Check sheet for the modelled part. Datum: model origin and axes. Units: mm. A direction names the side the tool comes from. Give positions to 0.01 mm unless a question says otherwise; leave off trailing zeros. Order: outer loops, then holes, each group sorted by start corner. A loop starts at its lowest first (then second) coordinate and runs counter-clockwise, first axis right, second up.
```python
from build123d import *

# Parameters (mm, degrees)
CYLINDER004_R     = 1.375
CYLINDER004_DEPTH = 4.7
CYLINDER005_R     = 1.375
CYLINDER005_DEPTH = 4.7
CYLINDER006_R     = 1.375
CYLINDER006_DEPTH = 4.7
CYLINDER007_R     = 1.375
CYLINDER007_DEPTH = 4.7
CYLINDER_R        = 2
CYLINDER_DEPTH    = 3
CYLINDER001_R     = 2
CYLINDER001_DEPTH = 3
CYLINDER002_R     = 2
CYLINDER002_DEPTH = 3
CYLINDER003_R     = 2
CYLINDER003_DEPTH = 3
BOX_W             = 100
BOX_H             = 100
BOX_DEPTH         = 3
CHAMFER_SIZE      = 1


with BuildPart() as main_ata_board_mounting_screws:
    # Cylinder004 → Cylinder004 (new body)
    with BuildSketch(Plane(origin=(8.3, 18.9, 3), x_dir=(1, 0, 0), z_dir=(0, 0, 1))):
        Circle(CYLINDER004_R)
    extrude(amount=CYLINDER004_DEPTH)


with BuildPart() as main_ata_board_mounting_screws001:
    # Cylinder005 → Cylinder005 (new body)
    with BuildSketch(Plane(origin=(8.3, 84.2, 3), x_dir=(1, 0, 0), z_dir=(0, 0, 1))):
        Circle(CYLINDER005_R)
    extrude(amount=CYLINDER005_DEPTH)


with BuildPart() as main_ata_board_mounting_screws002:
    # Cylinder006 → Cylinder006 (new body)
    with BuildSketch(Plane(origin=(89.6, 19, 3), x_dir=(1, 0, 0), z_dir=(0, 0, 1))):
        Circle(CYLINDER006_R)
    extrude(amount=CYLINDER006_DEPTH)


with BuildPart() as ata_board_mounting_screw_stubs:
    # Cylinder007 → Cylinder007 (new body)
    with BuildSketch(Plane(origin=(94.5, 82.2, 3), x_dir=(1, 0, 0), z_dir=(0, 0, 1))):
        Circle(CYLINDER007_R)
    extrude(amount=CYLINDER007_DEPTH)

    # Fusion001: union Main ATA Board Mounting Screws, Main ATA Board Mounting Screws001, Main ATA Board Mounting Screws002
    add(main_ata_board_mounting_screws.part)
    add(main_ata_board_mounting_screws001.part)
    add(main_ata_board_mounting_screws002.part)


with BuildPart() as f_1u_post_holes:
    # Cylinder → Cylinder (new body)
    with BuildSketch(Plane(origin=(6.5, 6.5, 0), x_dir=(1, 0, 0), z_dir=(0, 0, 1))):
        Circle(CYLINDER_R)
    extrude(amount=CYLINDER_DEPTH)


with BuildPart() as f_1u_post_holes001:
    # Cylinder001 → Cylinder001 (new body)
    with BuildSketch(Plane(origin=(93.5, 6.5, 0), x_dir=(1, 0, 0), z_dir=(0, 0, 1))):
        Circle(CYLINDER001_R)
    extrude(amount=CYLINDER001_DEPTH)


with BuildPart() as f_1u_post_holes002:
    # Cylinder002 → Cylinder002 (new body)
    with BuildSketch(Plane(origin=(93.5, 93.5, 0), x_dir=(1, 0, 0), z_dir=(0, 0, 1))):
        Circle(CYLINDER002_R)
    extrude(amount=CYLINDER002_DEPTH)


with BuildPart() as f_1u_post_holes_assembly:
    # Cylinder003 → Cylinder003 (new body)
    with BuildSketch(Plane(origin=(6.5, 93.5, 0), x_dir=(1, 0, 0), z_dir=(0, 0, 1))):
        Circle(CYLINDER003_R)
    extrude(amount=CYLINDER003_DEPTH)

    # Fusion: union 1U Post Holes, 1U Post Holes001, 1U Post Holes002
    add(f_1u_post_holes.part)
    add(f_1u_post_holes001.part)
    add(f_1u_post_holes002.part)


with BuildPart() as mounting_ata_aluminium:
    # Box → Box (new body)
    with BuildSketch(Plane.XY):
        with Locations((50, 50)):
            Rectangle(BOX_W, BOX_H)
    extrude(amount=BOX_DEPTH)

    # Cut: cut 1U post holes assembly
    add(f_1u_post_holes_assembly.part, mode=Mode.SUBTRACT)

    # Chamfer
    chamfer_edges = [mounting_ata_aluminium.edges().sort_by_distance(p)[0] for p in [
        (0, 0, 1.5),
        (0, 100, 1.5),
        (100, 0, 1.5),
        (100, 100, 1.5),
    ]]
    chamfer(chamfer_edges, length=CHAMFER_SIZE)

    # Fusion002: union ATA Board mounting screw stubs
    add(ata_board_mounting_screw_stubs.part)


with BuildPart() as mounting_ata_aluminium_1:
    # Fusion002 placement: moved
    add(mounting_ata_aluminium.part.moved(Location((0, 0, -3))))


solid = mounting_ata_aluminium_1.part
```
(1) Cross-section at B-B on z = 3.5. Enter the section's corners in (x, y) (3 decimals).
Response values:
outline: circle Ø2.75 at (8.3, 18.9); circle Ø2.75 at (8.3, 84.2); circle Ø2.75 at (89.6, 19); circle Ø2.75 at (94.5, 82.2)
(2) Set-up check for faces 4 (the face through (8.93, 17.68, 2.32)), 5 (the face through (49, 51, -3)): record each of +Z, -Z, +X, -X, +Y, -Y from which the full face is reachable in a straight line by a thin tool's end or side.
Response values:
face 4: +Z
face 5: -Z, +X, -X, +Y, -Y
(3) Gauge pin test, flat ends, axial feed: pin 1 Ø6 at (x, y) = (65.5, 11) entering from +Z; pin 2 Ø3 at (y, z) = (13.5, 0.5) entering from +X. Record the tip position at first contact, or that the pin passes through.
Response values:
pin 1: stops at z = 0
pin 2: stops at x = 100
(4) Cross-section at A-A on y = 6.5. Enter the section's corners in (x, z).
Response values:
outline: (0, -3) - (4.5, -3) - (4.5, 0) - (0, 0) - close; (8.5, -3) - (91.5, -3) - (91.5, 0) - (8.5, 0) - close; (95.5, -3) - (100, -3) - (100, 0) - (95.5, 0) - close
(5) Release check for a two-part mould opening along Y. For faces 1 (the face through (90, 19, 4.7)), 2 (the face through (88.587, 19.929, 2.317)), 3 (the face through (95.408, 7.101, -1.521)) record: released by +Y, released by -Y, zero draft, split by the parting line, or undercut.
Response values:
face 1: zero draft
face 2: split by the parting line
face 3: undercut
(6) Material ranges on L1, parallel to Y at x = 6.5, z = -2; L2, parallel to X at y = 92, z = -0.5; L3, parallel to Z at x = 84, y = 24.5, recorded low to high.
Response values:
L1: y = 0 to 4.5, 8.5 to 91.5, 95.5 to 100
L2: x = 0 to 5.18, 7.82 to 92.18, 94.82 to 100
L3: z = -3 to 0
(7) Cross-section at C-C on y = 32.5. Enter the section's corners in (x, z).
Response values:
outline: (0, -3) - (100, -3) - (100, 0) - (0, 0) - close
